```python
from build123d import *

# Parameters (mm, degrees)
DODANIE_WYCI_GNI_CIE1_DEPTH = 26
SZKIC2_W                    = 4.8
SZKIC2_H                    = 26
DODANIE_WYCI_GNI_CIE2_DEPTH = 5.5
ZAOKR_GLENIE1_R             = 0.75
SZKIC6_R                    = 1.6
WYTNIJ_WYCI_GNI_CIE3_DEPTH  = 2.5
SZKIC7_W                    = 6
SZKIC7_H                    = 16
WYTNIJ_WYCI_GNI_CIE4_DEPTH  = 2.4
SZKIC8_R                    = 1.6
WYTNIJ_WYCI_GNI_CIE5_DEPTH  = 2
ZAOKR_GLENIE2_R             = 0.6


with BuildPart() as part:
    # Szkic1 → Dodanie-wyciągnięcie1 (new body)
    with BuildSketch(Plane.XY):
        with BuildLine():
            Line((-6.75, -3.269174208), (-6.75, -7.242064623))
            ThreePointArc((-6.75, -7.242064623), (-9.078408451, -3.948733974), (-9.9, 0))
            Line((-9.9, 0), (-9.9, 15.5))
            Line((-9.9, 15.5), (9.9, 15.5))
            Line((9.9, 15.5), (9.9, 0))
            ThreePointArc((9.9, 0), (9.078408451, -3.948733974), (6.75, -7.242064623))
            Line((6.75, -7.242064623), (6.75, -3.269174208))
            ThreePointArc((6.75, -3.269174208), (0, 7.5), (-6.75, -3.269174208))
        make_face()
    extrude(amount=DODANIE_WYCI_GNI_CIE1_DEPTH)

    # Szkic2 → Dodanie-wyciągnięcie2 (add)
    with BuildSketch(Plane(origin=(0, 15.5, 0), x_dir=(1, 0, 0), z_dir=(0, 1, 0))):
        with Locations((-7.5, -13)):
            Rectangle(SZKIC2_W, SZKIC2_H)
        with Locations((7.5, -13)):
            Rectangle(SZKIC2_W, SZKIC2_H)
    extrude(amount=DODANIE_WYCI_GNI_CIE2_DEPTH)

    # Zaokrąglenie1
    zaokr_glenie1_edges = [part.edges().sort_by_distance(p)[0] for p in [
        (-6.75, -7.242064623, 13),
        (6.75, -7.242064623, 13),
    ]]
    fillet(zaokr_glenie1_edges, radius=ZAOKR_GLENIE1_R)

    # Szkic6 → Wytnij-wyciągnięcie3 (cut)
    with BuildSketch(Plane(origin=(0, 15.5, 0), x_dir=(1, 0, 0), z_dir=(0, 1, 0))):
        with Locations(Location((0, -13, 0), (0, 0, 180))):
            Circle(SZKIC6_R)
    extrude(amount=-WYTNIJ_WYCI_GNI_CIE3_DEPTH, mode=Mode.SUBTRACT)

    # Szkic7 → Wytnij-wyciągnięcie4 (cut)
    with BuildSketch(Plane(origin=(0, 13, 0), x_dir=(1, 0, 0), z_dir=(0, 1, 0))):
        with Locations((0, -8)):
            Rectangle(SZKIC7_W, SZKIC7_H)
    extrude(amount=-WYTNIJ_WYCI_GNI_CIE4_DEPTH, mode=Mode.SUBTRACT)

    # Szkic8 → Wytnij-wyciągnięcie5 (cut)
    with BuildSketch(Plane(origin=(0, 10.6, 0), x_dir=(1, 0, 0), z_dir=(0, 1, 0))):
        with Locations(Location((0, -13, 0), (0, 0, 180))):
            Circle(SZKIC8_R)
    extrude(amount=-WYTNIJ_WYCI_GNI_CIE5_DEPTH, mode=Mode.SUBTRACT)

    # Zaokrąglenie2
    zaokr_glenie2_edges = [part.edges().sort_by_distance(p)[0] for p in [
        (-5.1, 21, 13),
        (-9.9, 21, 13),
        (5.1, 21, 13),
        (9.9, 21, 13),
    ]]
    fillet(zaokr_glenie2_edges, radius=ZAOKR_GLENIE2_R)


solid = part.part
```
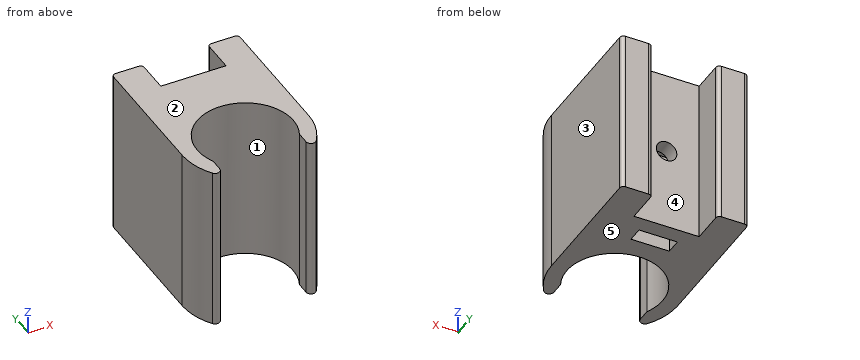
Geometry: final body of the model. Coordinates: model frame, mm. Face numbers are marked on the shaded views. A direction names the side the tool comes from. Coordinates: 2 decimals unless noted, no trailing zeros. Order: outer loops, then holes, each group sorted by start corner. A loop starts at its lowest first (then second) coordinate and runs counter-clockwise, first axis right, second up. Notation, with made-up numbers: M 59,89.5 L 95,89.5 A32 ccw 95,120.5 Z; hole C 65.25,68.5 d11. An arc over 180 degrees is marked long. Answer as CSV lines item,"result".
Q1. Section B-B on y = 17.5. Return the cut outline in (x, z), and give its area (3 significant figures).
Answers:
outline,"M -9.9,0 L -5.1,0 L -5.1,26 L -9.9,26 Z; M 5.1,0 L 9.9,0 L 9.9,26 L 5.1,26 Z"
area,"250 mm^2"
Q2. Line query: probe 1 along Z at (x, y) = (0, 13.5); probe 2 along X at (y, z) = (17.25, 9); probe 3 along X at (y, z) = (2, 20.5). Output: solid intervals per line, ascending. Write a range as [from, to].
Answers:
probe 1,"z = [0, 11.4], [14.6, 26]"
probe 2,"x = [-9.9, -5.1], [5.1, 9.9]"
probe 3,"x = [-9.9, -7.23], [7.23, 9.9]"
Q3. First-contact query: P1, Ø1, axis at x = 0.5, z = 12.5, coming from the +Y side; P2, Ø2, axis at x = -2.5, z = 14.5, coming from the +Y side; P3, Ø1, axis at x = -1.5, z = 3.5, coming from the -Y side. Flat tips, straight axial feed; report the tip coordinate or a pass-through.
Answers:
P1,"stops at y = 8.6"
P2,"stops at y = 15.5"
P3,"stops at y = 7.23"
Q4. Set-up query: the marked faces 4 and 5. Return all of +Z, -Z, +X, -X, +Y, -Y with unobstructed straight access to the full face (end or side cutting, diameter ignored); none if empty.
Answers:
face 4,"+Z, -Z, +Y"
face 5,"-Z, +X, -X, +Y, -Y"
Q5. Section C-C on z = 8. Return the cut outline in (x, y), and give its area (3 significant figures).
Answers:
outline,"M -9.9,0 A9.9 ccw -8.11,-5.67 A0.75 ccw -6.75,-5.24 L -6.75,-3.27 A7.5 cw long 6.75,-3.27 L 6.75,-5.24 A0.75 ccw 8.11,-5.67 A9.9 ccw 9.9,0 L 9.9,20.4 A0.6 ccw 9.3,21 L 5.7,21 A0.6 ccw 5.1,20.4 L 5.1,15.5 L -5.1,15.5 L -5.1,20.4 A0.6 ccw -5.7,21 L -9.3,21 A0.6 ccw -9.9,20.4 Z; hole M -3,10.6 L 3,10.6 L 3,13 L -3,13 Z"
area,"283 mm^2"
Q6. Draft query along X for the marked faces 1, 2 and 3. Return one class per face: pulls with the +X half, pulls with the -X half, needs draft (parallel to the pull), parting line crosses it, or undercut.
Answers:
face 1,"undercut"
face 2,"needs draft"
face 3,"pulls with the +X half"
Q7. Section A-A on x = 0. Return the cut outline in (y, z), and give its area (3 significant figures).
Answers:
outline,"M 7.5,0 L 10.6,0 L 10.6,11.4 L 8.6,11.4 L 8.6,14.6 L 10.6,14.6 L 10.6,16 L 13,16 L 13,14.6 L 15.5,14.6 L 15.5,26 L 7.5,26 Z; M 13,0 L 15.5,0 L 15.5,11.4 L 13,11.4 Z"
area,"155 mm^2"
